Here's the drawing with two shaded views (mm, measured from the low corner). I have some questions. Round coordinates to 2 decimals unless told otherwise and drop trailing zeros. Loops run counter-clockwise (first coordinate to the right, second up) from the corner with the lowest first, then second, coordinate; pieces in that order, holes last. Notation, with made-up numbers: (70, 33) -> (114, 33) arc R30 ccw to (114, 69) -> close; hole circle Ø2 at (19, 74). An arc over 180 degrees is marked (long way). Write item = value, one per line.
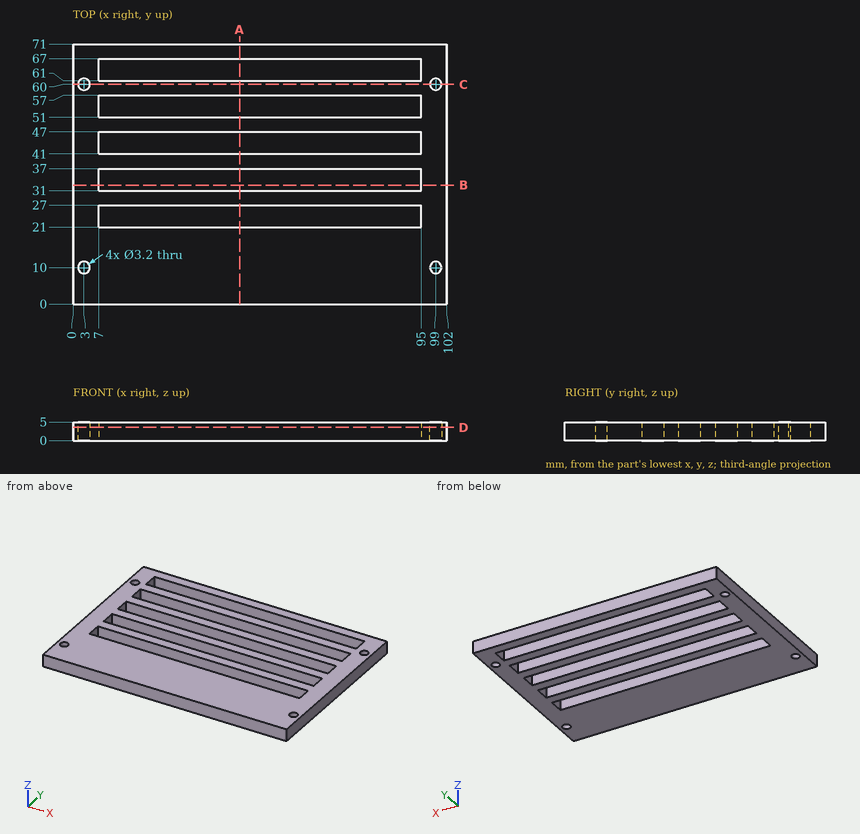
1. Suppose I cut it at B-B, the plane y = 32.5. List the corners of the cut face in (x, z) for me.
Entries:
outline = (0, 0) -> (7, 0) -> (7, 5) -> (0, 5) -> close; (95, 0) -> (102, 0) -> (102, 5) -> (95, 5) -> close
2. Suppose I cut it at A-A, the plane x = 45.5. List the corners of the cut face in (y, z) for me, and give its area (3 significant figures).
Entries:
outline = (0, 0) -> (21, 0) -> (21, 5) -> (0, 5) -> close; (27, 0) -> (31, 0) -> (31, 5) -> (27, 5) -> close; (37, 0) -> (41, 0) -> (41, 5) -> (37, 5) -> close; (47, 0) -> (51, 0) -> (51, 5) -> (47, 5) -> close; (57, 0) -> (61, 0) -> (61, 5) -> (57, 5) -> close; (67, 0) -> (71, 0) -> (71, 5) -> (67, 5) -> close
area = 205 mm²
3. Suppose I cut it at C-C, the plane y = 60. List the corners of the cut face in (x, z) for me, and give its area (3 significant figures).
Entries:
outline = (0, 0) -> (1.4, 0) -> (1.4, 5) -> (0, 5) -> close; (4.6, 0) -> (97.4, 0) -> (97.4, 5) -> (4.6, 5) -> close; (100.6, 0) -> (102, 0) -> (102, 5) -> (100.6, 5) -> close
area = 478 mm²
4. I need wall thicknesses on line 1 (Y direction, x = 54.5, z = 0.9); line 2 (Y direction, x = 99, z = 1.9); line 3 (X direction, y = 36, z = 1.3). Which ranges of each line are inside material? Lowest first, please. Write a range as [from, to].
Entries:
line_1 = [0, 21], [27, 31], [37, 41], [47, 51], [57, 61], [67, 71]
line_2 = [0, 8.4], [11.6, 58.4], [61.6, 71]
line_3 = [0, 7], [95, 102]
5. Suppose I cut it at D-D, the plane z = 3.6. Count the separate pieces of the cut face and the enclosed holes in it, and give its area (3 significant figures).
Entries:
separate_pieces = 1
enclosed_holes = 9
area = 4,570 mm²
